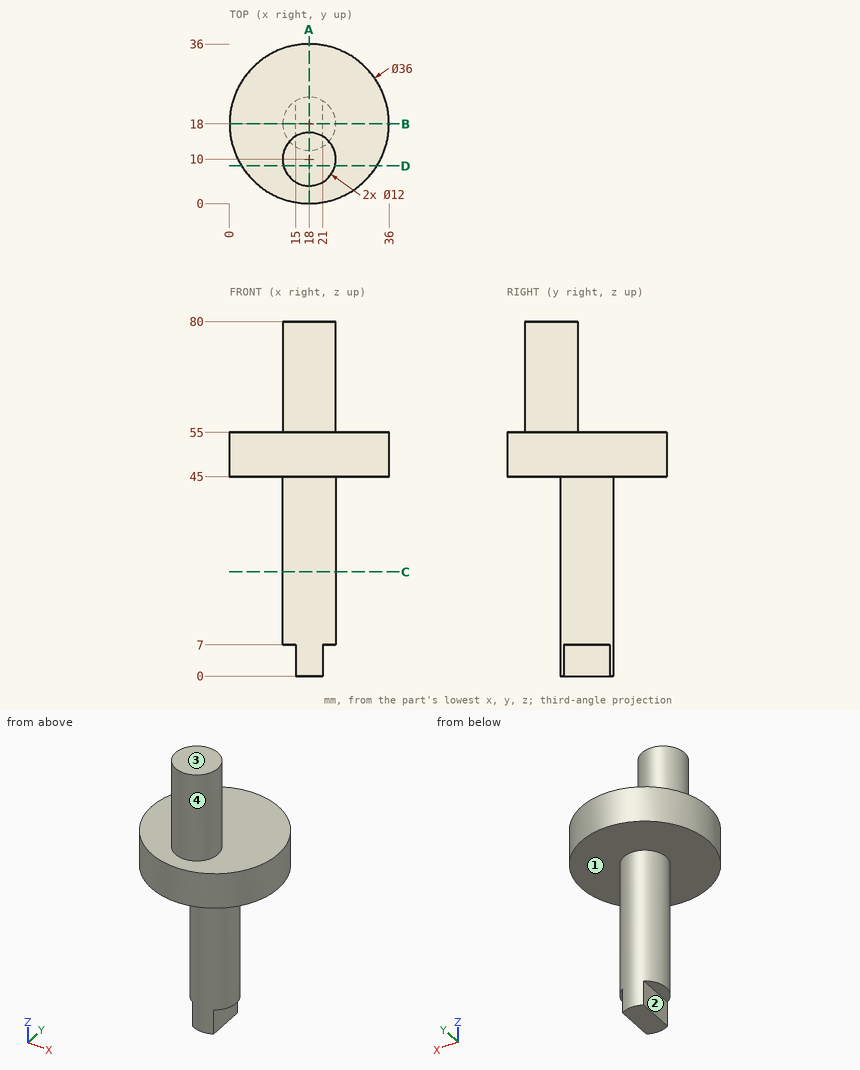
For this review, use the dimensioned drawing (mm, ordinates from the lowest corner) and the shaded views. A direction names the side the tool comes from. Round coordinates to 2 decimals unless told otherwise and drop trailing zeros. Write each loop counter-clockwise with the first axis right and the second up, starting at its lowest first coordinate (ties: lowest second). Pieces come first, ordered by that corner, then holes. Notation, with made-up numbers: (58.5, -28.75) - (89.5, -28.75) arc R18 ccw to (89.5, -22.75) - close; hole circle Ø1 at (42, 34.25). An arc over 180 degrees is marked (long way). Answer as a JSON object with one key per item and string values.
1. We need section B-B on y = 18. Give the boundary of the cut face in (x, z), then the cut area to 3 significant figures.
Response values:
{"outline": "(0, 45) - (12, 45) - (12, 7) - (15, 7) - (15, 0) - (21, 0) - (21, 7) - (24, 7) - (24, 45) - (36, 45) - (36, 55) - (0, 55) - close", "area": "858 mm2"}
2. We need section C-C on z = 23.5. Give the boundary of the cut face in (x, y).
Response values:
{"outline": "circle Ø12 at (18, 18)"}
3. Tool access review of the marked faces 1, 2, 3 and 4: name each direction out of +Z, -Z, +X, -X, +Y, -Y from which nothing blocks a thin tool from reaching the whole face with its end or side.
Response values:
{"face 1": "-Z", "face 2": "-Z, -X, +Y, -Y", "face 3": "+Z, +X, -X, +Y, -Y", "face 4": "+Z"}
4. To check wall thickness, follow line 1 along Z through (x, y) = (13, 18); line 2 along Z through (x, y) = (26.5, 13.5); line 3 along X through (y, z) = (21, 28). State the ranges of each line that lie inside material, in increasing order.
Response values:
{"line 1": "z = 7 to 55", "line 2": "z = 45 to 55", "line 3": "x = 12.8 to 23.2"}
5. We need section A-A on x = 18. Give the boundary of the cut face in (y, z).
Response values:
{"outline": "(0, 45) - (12, 45) - (12, 0) - (24, 0) - (24, 45) - (36, 45) - (36, 55) - (16, 55) - (16, 80) - (4, 80) - (4, 55) - (0, 55) - close"}
6. We need section D-D on y = 8.5. Give the boundary of the cut face in (x, z).
Response values:
{"outline": "(2.71, 45) - (33.29, 45) - (33.29, 55) - (23.81, 55) - (23.81, 80) - (12.19, 80) - (12.19, 55) - (2.71, 55) - close"}
7. For pin 1 Ø2 at (y, z) = (16, 4.5) entering from -X; pin 2 Ø4 at (x, z) = (22, 21.5) entering from -Y; pin 3 Ø1 at (y, z) = (21.5, 40.5) entering from +X, all flat-tipped, find the tip position at first contact; note any pin that passes through.
Response values:
{"pin 1": "stops at x = 15", "pin 2": "stops at y = 12.34", "pin 3": "stops at x = 23.2"}
